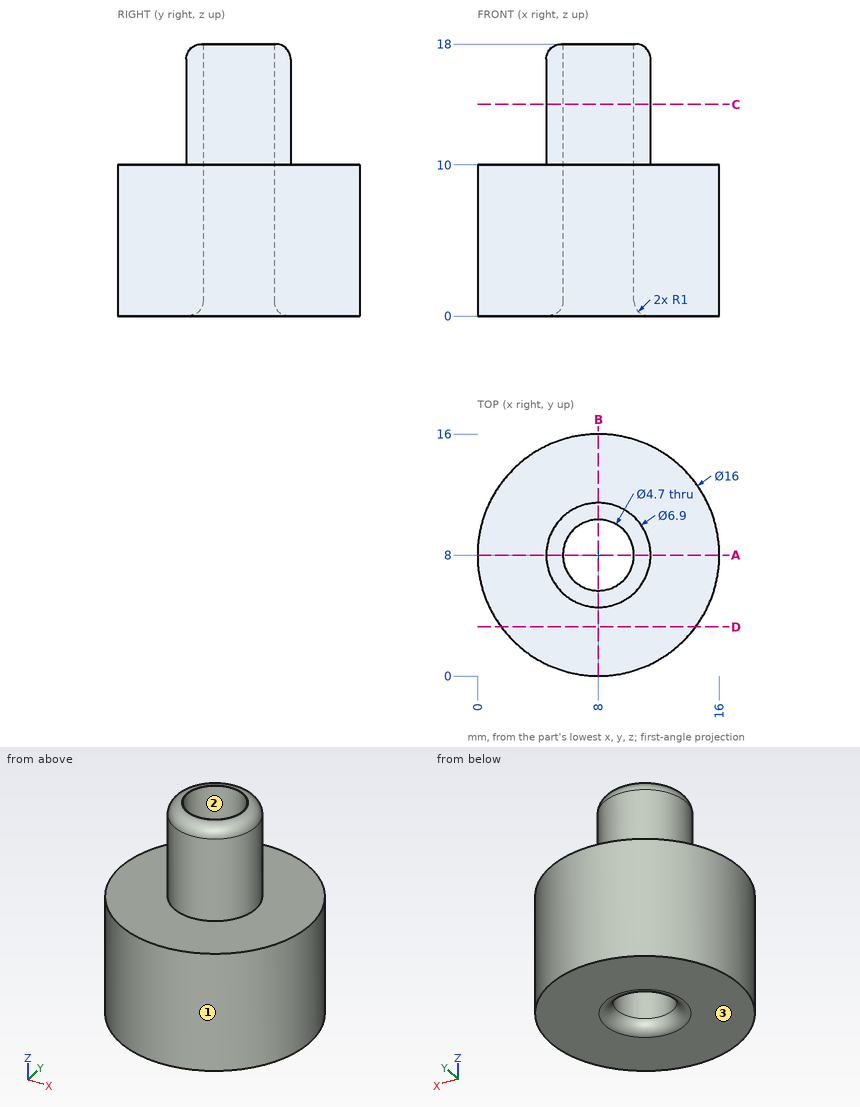
Source: three-view drawing plus pictorial views. Frame: mm from the lowest corner of the part. Coordinates: 2 decimals unless noted, no trailing zeros. Loops run counter-clockwise (first coordinate to the right, second up) from the corner with the lowest first, then second, coordinate; pieces in that order, holes last. Notation, with made-up numbers: (23, 4) -> (44, 4) arc R28 ccw to (44, 30) -> close; hole circle Ø8 at (74.5, 41). An arc over 180 degrees is marked (long way). One line per item, written item: value.
(1) Ray query, line 1 along Y through (x, z) = (8, 13); line 2 along Y through (x, z) = (8, 8.5); line 3 along Z through (x, y) = (11.25, 10.5). Return the intervals inside material, ascending.
Answer below:
line 1: y = 4.55 to 5.65, 10.35 to 11.45
line 2: y = 0 to 5.65, 10.35 to 16
line 3: z = 0 to 10
(2) Draft query along Y for the marked faces 1, 2 and 3. Return one class per face: pulls with the +Y half, pulls with the -Y half, needs draft (parallel to the pull), parting line crosses it, or undercut.
Answer below:
face 1: parting line crosses it
face 2: undercut
face 3: needs draft
(3) Cut plane C-C (z = 14). Output: boundary loops of the cut face in (x, y), then the cut area to 3 significant figures.
Answer below:
outline: circle Ø6.9 at (8, 8); hole circle Ø4.7 at (8, 8)
area: 20.0 mm2
(4) Pin query (flat end, axial travel): pin 1 Ø4 at (x, z) = (9, 15) entering from +Y; pin 2 Ø5 at (y, z) = (11, 14.5) entering from -X; pin 3 Ø5.5 at (x, y) = (8, 8) entering from -Z. Return the tip coordinate at first contact, or that it passes through.
Answer below:
pin 1: stops at y = 11.45
pin 2: stops at x = 4.59
pin 3: stops at z = 0.2
(5) Cut plane D-D (y = 3.25). Output: boundary loops of the cut face in (x, z).
Answer below:
outline: (1.56, 0) -> (14.44, 0) -> (14.44, 10) -> (1.56, 10) -> close
(6) Cut plane A-A (y = 8). Output: boundary loops of the cut face in (x, z).
Answer below:
outline: (0, 0) -> (4.65, 0) arc R1 ccw to (5.65, 1) -> (5.65, 18) -> (5.55, 18) arc R1 ccw to (4.55, 17) -> (4.55, 10) -> (0, 10) -> close; (10.35, 1) arc R1 ccw to (11.35, 0) -> (16, 0) -> (16, 10) -> (11.45, 10) -> (11.45, 17) arc R1 ccw to (10.45, 18) -> (10.35, 18) -> close
